```python
from build123d import *

# Parameters (mm, degrees)
F0_R     = 40
F1_DEPTH = 30
F2_DEPTH = 15
F3_DEPTH = 25


with BuildPart() as f1:
    # F0 (on Front) → F1 (new body, symmetric)
    with BuildSketch(Plane.XZ):
        with BuildLine():
            ThreePointArc((80, 25), (58.736468, 28.697259), (41.012193, 41.012193))
            ThreePointArc((41.012193, 41.012193), (10.882045, 56.970002), (-23.008546, 53.241026))
            ThreePointArc((-23.008546, 53.241026), (-47.67685, -33.029047), (41.759702, -40.250805))
            ThreePointArc((41.759702, -40.250805), (59.237365, -28.506986), (80, -25))
            Line((80, -25), (170, -25))
            ThreePointArc((170, -25), (193.856579, -7.474199), (184.264706, 20.530908))
            ThreePointArc((184.264706, 20.530908), (177.474199, 23.856579), (170, 25))
            Line((170, 25), (80, 25))
        make_face()
        Circle(F0_R, mode=Mode.SUBTRACT)
        with BuildLine():
            ThreePointArc((80, -12.5), (67.5, 0), (80, 12.5))
            Line((80, 12.5), (170, 12.5))
            ThreePointArc((170, 12.5), (182.5, 0), (170, -12.5))
            Line((170, -12.5), (80, -12.5))
        make_face(mode=Mode.SUBTRACT)
    extrude(amount=F1_DEPTH, both=True)

    # F0 (on Front) → F2 (join, symmetric)
    with BuildSketch(Plane.XZ):
        with BuildLine():
            ThreePointArc((-23.008546, 53.241026), (10.882045, 56.970002), (41.012193, 41.012193))
            ThreePointArc((41.012193, 41.012193), (58.736468, 28.697259), (80, 25))
            Line((80, 25), (170, 25))
            ThreePointArc((170, 25), (177.474199, 23.856579), (184.264706, 20.530908))
            Line((184.264706, 20.530908), (69.611765, 100.190829))
            ThreePointArc((69.611765, 100.190829), (78.249713, 93.60012), (86.267027, 86.267027))
            ThreePointArc((86.267027, 86.267027), (86.267027, 55.154329), (55.154329, 55.154329))
            ThreePointArc((55.154329, 55.154329), (29.849308, 72.062604), (0, 78))
            ThreePointArc((0, 78), (-8.852226, 79.859541), (-16.207991, 85.12381))
            ThreePointArc((-16.207991, 85.12381), (-11.382532, 67.427879), (-23.008546, 53.241026))
        make_face()
    extrude(amount=F2_DEPTH, both=True)

    # F0 (on Front) → F3 (join, symmetric)
    with BuildSketch(Plane.XZ):
        with BuildLine():
            ThreePointArc((0, 122), (-20.140459, 108.852226), (-16.207991, 85.12381))
            ThreePointArc((-16.207991, 85.12381), (-8.852226, 79.859541), (0, 78))
            ThreePointArc((0, 78), (29.849308, 72.062604), (55.154329, 55.154329))
            ThreePointArc((55.154329, 55.154329), (86.267027, 55.154329), (86.267027, 86.267027))
            ThreePointArc((86.267027, 86.267027), (78.249713, 93.60012), (69.611765, 100.190829))
            ThreePointArc((69.611765, 100.190829), (36.474093, 116.420104), (0, 122))
        make_face()
        with BuildLine():
            ThreePointArc((0, 109), (41.712494, 100.702869), (77.074639, 77.074639))
            ThreePointArc((77.074639, 77.074639), (77.074639, 64.346717), (64.346717, 64.346717))
            ThreePointArc((64.346717, 64.346717), (34.824192, 84.073037), (0, 91))
            ThreePointArc((0, 91), (-9, 100), (0, 109))
        make_face(mode=Mode.SUBTRACT)
    extrude(amount=F3_DEPTH, both=True)


solid = f1.part
```
Input: part model. Units: mm. Frame: model coordinates. A direction names the side the tool comes from. Give positions to 0.01 mm unless a question says otherwise; leave off trailing zeros. Order: outer loops, then holes, each group sorted by start corner. A loop starts at its lowest first (then second) coordinate and runs counter-clockwise, first axis right, second up. Notation, with made-up numbers: M 56,-3.75 L 91,-3.75 A22 cw 91,29.25 Z; hole C -3.5,51 d3. An arc over 180 degrees is marked long. Return JSON: item names as keys, results as strings.
1) Section query C-C on x = 24.5. Output: boundary loops of the cut face in (y, z), and give its area (3 significant figures).
Taken from the geometry:
{"outline": "M -30,-52.57 L 30,-52.57 L 30,-31.62 L -30,-31.62 Z; M -30,31.62 L 30,31.62 L 30,52.57 L 15,52.57 L 15,74.05 L 25,74.05 L 25,87.64 L -25,87.64 L -25,74.05 L -15,74.05 L -15,52.57 L -30,52.57 Z; M -25,106.21 L 25,106.21 L 25,119.51 L -25,119.51 Z", "area": "4,500 mm2"}
2) Access query for faces 4 (the face through (80, -15, 46)), 5 (the face through (-9, 0, 100)), 6 (the face through (78.37, 19.93, 93.5)), 7 (the face through (85.921, 19.93, 54.816)). Directions: +Z, -Z, +X, -X, +Y, -Y. A direction counts if a zero-diameter tool reaches every point of the face in a straight line with its end or side. Return the directions, or none.
Taken from the geometry:
{"face 4": "-Y", "face 5": "+Y, -Y", "face 6": "+Z, +X, +Y", "face 7": "+Y"}
3) Section query A-A on z = 0. Output: boundary loops of the cut face in (x, y), and give its area (3 significant figures).
Taken from the geometry:
{"outline": "M -58,-30 L -40,-30 L -40,30 L -58,30 Z; M 40,-30 L 67.5,-30 L 67.5,30 L 40,30 Z; M 182.5,-30 L 195,-30 L 195,30 L 182.5,30 Z", "area": "3,480 mm2"}
4) Section query B-B on y = 9. Output: boundary loops of the cut face in (x, z).
Taken from the geometry:
{"outline": "M -23.01,53.24 A58 ccw long 41.76,-40.25 A50 cw 80,-25 L 170,-25 A25 ccw 184.26,20.53 L 69.61,100.19 A122 ccw 0,122 A22 ccw -16.21,85.12 A20 cw Z; hole C 0,0 d80; hole M 0,91 A91 cw 64.35,64.35 A9 ccw 77.07,77.07 A109 ccw 0,109 A9 ccw Z; hole M 80,-12.5 L 170,-12.5 A12.5 ccw 170,12.5 L 80,12.5 A12.5 ccw Z"}
5) Mould query, pull axis Z, two halves, no side actions, for faces 1 (the face through (29.453, -20.07, 72.226)), 2 (the face through (39, 30, -12)), 3 (the face through (78.37, -20.07, 93.5)). Classes: released by +Z, released by -Z, zero draft, split by the parting line, or undercut.
Taken from the geometry:
{"face 1": "undercut", "face 2": "zero draft", "face 3": "released by +Z"}
6) Contact query for flat-ended pins moving along their axis: pin 1 (3 mm diameter, centred on x = 149, z = 42.5, fed in from -Y); pin 2 (12 mm diameter, centred on x = 126.5, y = -23.5, fed in from +Z); pin 3 (6 mm diameter, centred on x = -16.5, y = 5.5, fed in from -Z). Output: stop coordinate, or through.
Taken from the geometry:
{"pin 1": "stops at y = -15", "pin 2": "stops at z = 25", "pin 3": "stops at z = -56.41"}
7) Section query D-D on x = 126. Output: boundary loops of the cut face in (y, z).
Taken from the geometry:
{"outline": "M -30,-25 L 30,-25 L 30,-12.5 L -30,-12.5 Z; M -30,12.5 L 30,12.5 L 30,25 L 15,25 L 15,61.01 L -15,61.01 L -15,25 L -30,25 Z"}
8) Line query: L1, parallel to Z at x = 1.5, y = -5.5; L2, parallel to Z at x = 170, y = -26; L3, parallel to Y at x = 48, z = 48. Output: solid intervals per line, ascending. Write a range as [from, to].
Taken from the geometry:
{"L1": "z = [-57.98, -39.97], [39.97, 90.99], [108.99, 121.99]", "L2": "z = [-25, -12.5], [12.5, 25]", "L3": "y = [-15, 15]"}
